```python
from build123d import *

# Parameters (mm, degrees)
F1_DEPTH = 50


with BuildPart() as f1:
    # F0 (on Front) → F1 (new body)
    with BuildSketch(Plane.XZ):
        with BuildLine():
            Line((-78, 0), (-50, 0))
            ThreePointArc((-50, 0), (0, 50), (50, 0))
            Line((50, 0), (149.356318, 0))
            Line((149.356318, 0), (149.356318, 10))
            Line((149.356318, 10), (77.356318, 10))
            ThreePointArc((77.356318, 10), (0, 78), (-77.356318, 10))
            Line((-77.356318, 10), (-150.643682, 10))
            Line((-150.643682, 10), (-150.643682, 0))
            Line((-150.643682, 0), (-78, 0))
        make_face()
    extrude(amount=F1_DEPTH)


solid = f1.part
```
The listing builds one solid part. Answer for the finished solid, in the listing's coordinates (mm). A direction names the side the tool comes from. Coordinates: 2 decimals unless noted, no trailing zeros. Order: outer loops, then holes, each group sorted by start corner. A loop starts at its lowest first (then second) coordinate and runs counter-clockwise, first axis right, second up. Notation, with made-up numbers: M 83.25,59 L 104.25,59 A16 ccw 104.25,81 Z; hole C 11,-14 d5. An arc over 180 degrees is marked long. Answer as a JSON object with one key per item and string values. Group by question number.
1. Flat-ended cylindrical pins translate along their axes: P1, Ø1.5, axis at x = 3.5, y = -42.5, coming from the +Z side; P2, Ø25, axis at x = 96, y = -35.5, coming from the +Z side; P3, Ø1, axis at y = -20, z = 19.5, coming from the +X side. Find the tip coordinate at first contact, or state that the pin passes through.
2. Section D-D on z = 68 is taken. Write down the section's boundary in (x, y).
3. Section B-B on y = -43.5 is taken. Write down the section's boundary in (x, z), then the cut area to 3 significant figures.
4. A tool of negligible diameter and unlimited length cuts with its end or side. For faces 4 (the flat face through (114, -25, 10)), 5 (the flat face through (-113, -25, 10)), 6 (the flat face through (-1, -50, 54)), from which of +Z, -Z, +X, -X, +Y, -Y can it reach the whole face along a straight path? Write none if from no direction.
5. Determine the mould class of faces 1 (the cylindrical face through (-1.099, -24.65, 49.988)), 2 (the flat face through (-101, -25, 0)), 3 (the flat face through (-150.644, -25, 5)) for opening direction X: released by +X, released by -X, zero draft, split by the parting line, or undercut.
6. Section A-A on z = 45 is taken. Write down the section's boundary in (x, y).
7. Section C-C on x = 0 is taken. Write down the section's boundary in (y, z).
8. Straight lines are drawn through the part: line 1 (Z direction, x = -107, y = -5); line 2 (X direction, y = -7, z = 7); line 3 (X direction, y = -40, z = 22.5). For each, find the intervals that lie inside material, in ascending order.
Values follow:
{
 "1": {"P1": "z = 77.95", "P2": "z = 10", "P3": "x = 75.65"},
 "2": {"outline": "M -38.21,-50 L 38.21,-50 L 38.21,0 L -38.21,0 Z"},
 "3": {"outline": "M -150.64,0 L -50,0 A50 cw 50,0 L 149.36,0 L 149.36,10 L 77.36,10 A78 ccw -77.36,10 L -150.64,10 Z", "area": "7,070 mm2"},
 "4": {"face 4": "+Z, +X, +Y, -Y", "face 5": "+Z, -X, +Y, -Y", "face 6": "+Z, -Z, +X, -X, -Y"},
 "5": {"face 1": "undercut", "face 2": "zero draft", "face 3": "released by -X"},
 "6": {"outline": "M -63.71,-50 L -21.79,-50 L -21.79,0 L -63.71,0 Z; M 21.79,-50 L 63.71,-50 L 63.71,0 L 21.79,0 Z"},
 "7": {"outline": "M -50,50 L 0,50 L 0,78 L -50,78 Z"},
 "8": {"line 1": "0 to 10", "line 2": "-150.64 to -49.51, 49.51 to 149.36", "line 3": "-74.68 to -44.65, 44.65 to 74.68"}
}
